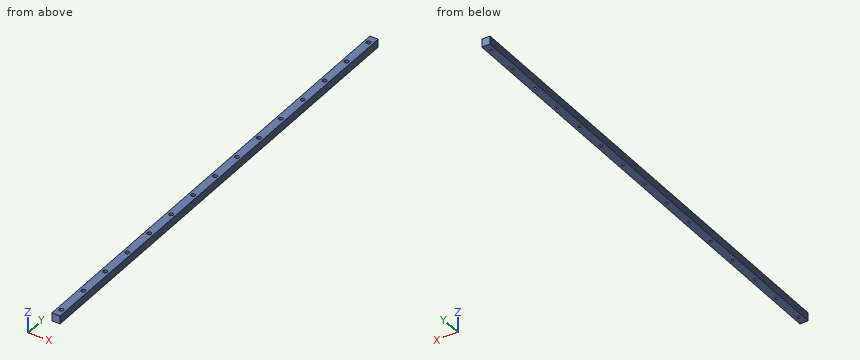
```python
from build123d import *

# Parameters (mm, degrees)
SKETCH_1_W                = 15
SKETCH_1_H                = 15
EXTRUDE_1_DEPTH           = 435
HOLE_WIZARD_1_D           = 4.5
HOLE_WIZARD_1_DEPTH       = 60
HOLE_WIZARD_1_CBORE_D     = 7.5
HOLE_WIZARD_1_CBORE_DEPTH = 5.3
PATTERN_LINEAR_1_COUNT    = 15
PATTERN_LINEAR_1_PITCH    = 60


with BuildPart() as part:
    # 草图1 → 凸台-拉伸1 (new, symmetric)
    with BuildSketch(Plane(origin=(0, 0, 0), x_dir=(1, 0, 0), z_dir=(0, 1, 0))):
        with Locations((0, -7.5)):
            Rectangle(SKETCH_1_W, SKETCH_1_H)
    extrude(amount=EXTRUDE_1_DEPTH, both=True)

    # 孔1
    with Locations(Plane.XY.offset(15)):
        with Locations((0, 420)):
            hole_wizard_1 = CounterBoreHole(HOLE_WIZARD_1_D / 2, HOLE_WIZARD_1_CBORE_D / 2, HOLE_WIZARD_1_CBORE_DEPTH, depth=HOLE_WIZARD_1_DEPTH)

    # 阵列(线性)1: 孔1 ×15
    with Locations(*[(0, -i * PATTERN_LINEAR_1_PITCH, 0) for i in range(1, PATTERN_LINEAR_1_COUNT)]):
        add(hole_wizard_1, mode=Mode.SUBTRACT)


solid = part.part
```
Design review of the part built by this model. Coordinates are the model's own, in mm. Give positions to 0.01 mm unless a question says otherwise; leave off trailing zeros. Return JSON: item names as keys, results as strings. Group by question number.
Item 1: We need section A-A (z = 5.5). Give the number of separate pieces and of enclosed holes in the cut face, and give its area (3 significant figures).
Item 2: Insertion check: pin 1 Ø3.5 at (x, y) = (0, -180) entering from +Z; pin 2 Ø6 at (x, y) = (0, -300) entering from -Z; pin 3 Ø2 at (x, y) = (-1.5, -179.5) entering from +Z. Each pin has a flat end and moves straight along its axis. Give the tip position at first contact, or say it passes through.
Item 3: For probe 1 along X at (y, z) = (360, 12.05); probe 2 along X at (y, z) = (-420, 7), list the stretches that pass through material, from the lowest coordinate up.
Output:
{
 "1": {"separate pieces": "1", "enclosed holes": "15", "area": "12,800 mm^2"},
 "2": {"pin 1": "passes through", "pin 2": "stops at z = 0", "pin 3": "stops at z = 9.7"},
 "3": {"probe 1": "x = -7.5 to -3.75, 3.75 to 7.5", "probe 2": "x = -7.5 to -2.25, 2.25 to 7.5"}
}
